Autodesk Inventor part; units mm, degrees
ref_plane "YZ Plane" through (0, 0, 0) normal (1, 0, 0) x (0, 1, 0)
ref_plane "XZ Plane" through (0, 0, 0) normal (0, 1, 0) x (-1, 0, 0)
ref_plane "XY Plane" through (0, 0, 0) normal (0, 0, 1) x (1, 0, 0)
sketch "Sketch1" plane through (0, 0, 0) normal (0, 0, 1) x (1, 0, 0)
  line L0 (0, 0) -> (400, 0)
  line L1 (400, 0) -> (400, 70.7107)
  line L2 (400, 70.7107) -> (-70.7107, 70.7107)
  line L3 (-70.7107, 70.7107) -> (0, 0) construction
  line L4 (0, 0) -> (-56.5685, -56.5685)
  line L5 (-56.5685, -56.5685) -> (-127.2792, 14.1421)
  line L6 (-127.2792, 14.1421) -> (-70.7107, 70.7107)
  dimension "d0" = 400
  dimension "d2" = 135
  dimension "d3" = 80
  dimension "d6" = 100
extrude "Extrusion1" add sketch "Sketch1" along normal blind 5
mirror "Mirror1" about plane through (-127.2792, 14.1421, 0) normal (-0.7071068, -0.7071068, 0)
properties part number "leg" material "Plywood, Finish"
Can you work these out from the model? Positions are in its coordinate system, mm. Round coordinates to 2 decimals unless told otherwise and drop trailing zeros. Loops run counter-clockwise (first coordinate to the right, second up) from the corner with the lowest first, then second, coordinate; pieces in that order, holes last. Notation, with made-up numbers: M -33.5,56 L 8.5,56 A17 ccw 8.5,84 Z; hole C -21,26 d7. An arc over 180 degrees is marked long. Answer in a Markdown table with one row per item.
1. If we section it at B-B, the plane y = -78: Please give me the cut outline in (x, z).
Established:
| item | result |
|---|---|
| outline | M -183.85,0 L -78,0 L -78,5 L -183.85,5 Z |
2. I'm going to push flat-ended pins straight in: pin 1 Ø1.5 at (x, z) = (-74, 1) entering from -Y; pin 2 Ø1.5 at (y, z) = (-221.5, 3.5) entering from +X. Where does each tip first touch, or does it pass through?
Established:
| item | result |
|---|---|
| pin 1 | y = -74.75 |
| pin 2 | x = -113.14 |
3. If we section it at A-A, the plane z = 4: Please give me the cut outline in (x, y), plus the area to 3 significant figures.
Established:
| item | result |
|---|---|
| outline | M -183.85,-513.14 L -113.14,-513.14 L -113.14,-113.14 L 0,0 L 400,0 L 400,70.71 L -70.71,70.71 L -127.28,14.14 L -183.85,-42.43 Z |
| area | 77,600 mm² |
4. Please list where these lines run through material, in increasing order: line 1 (Y direction, x = 229, z = 2.2); line 2 (X direction, y = -294.5, z = 3.25); line 3 (Y direction, x = -133, z = 3.1). Write a range as from..to.
Established:
| item | result |
|---|---|
| line 1 | 0..70.71 |
| line 2 | -183.85..-113.14 |
| line 3 | -513.14..8.42 |
5. If we section it at C-C, the plane x = 261: Please give me the cut outline in (y, z).
Established:
| item | result |
|---|---|
| outline | M 0,0 L 70.71,0 L 70.71,5 L 0,5 Z |
